```python
from build123d import *

# Parameters (mm, degrees)
F3_DEPTH        = 6
F3_COPIES_COUNT = 9


# Not quite as in the source:
# - a pattern or mirror of a feature is missing from the dataset's text; its kind, count and spacing are read off the source's solid


with BuildPart() as f1:
    # F0 (on Front) → F1 (revolve)
    with BuildSketch(Plane.XZ):
        Polygon((6, 0), (2.5, 0), (2, -2), (2, -10), (4.25, -10), (4.25, -4), (4.9, -4), (4.9, -2), (6, -2), align=None)
    revolve(axis=Axis((0, 0, -12.1953526796), (0, 0, -1)))

    # F2 (on face) → F3 (join, through all)
    with BuildSketch(Plane(origin=(0, 0, -10), x_dir=(1, 0, 0), z_dir=(0, 0, -1))):
        with BuildLine():
            ThreePointArc((-0.75, 4.1833001327), (0, 4.25), (0.75, 4.1833001327))
            Line((0.75, 4.1833001327), (0.75, 4.3833001327))
            Line((0.75, 4.3833001327), (-0.75, 4.3833001327))
            Line((-0.75, 4.3833001327), (-0.75, 4.1833001327))
        make_face()
    f3 = extrude(amount=-F3_DEPTH)

    # F3_copies: F3 ×9 about axis
    f3_copies_axis = Axis((0, 0, 0), (0, 0, 1))
    for i in range(1, F3_COPIES_COUNT):
        add(f3.rotate(f3_copies_axis, i * 360 / F3_COPIES_COUNT))


solid = f1.part
```
Can you work these out from the model? Positions are in its coordinate system, mm. A direction names the side the tool comes from. Coordinates: 2 decimals unless noted, no trailing zeros. Write each loop counter-clockwise with the first axis right and the second up, starting at its lowest first coordinate (ties: lowest second). Pieces come first, ordered by that corner, then holes. Notation, with made-up numbers: (-6.75, 79) - (-1.75, 79) arc R16 ccw to (-1.75, 86) - close; hole circle Ø10 at (64, 67.25). An arc over 180 degrees is marked (long way). Return JSON: item names as keys, results as strings.
Q1. If we section it at B-B (z = -1): Please give me the cut outline in (x, y), then the cut area to 3 significant figures.
Computed values:
{"outline": "circle Ø12 at (0, 0); hole circle Ø4.5 at (0, 0)", "area": "97.2 mm2"}
Q2. Thinking about a two-plate mould opening in X: for faces 4 (the cylindrical face through (1.46, -3.99, -6.96)), 5 (the cylindrical face through (4.184, 0.748, -6.958)), 6 (the flat face through (3, 0, 0)), which applies, +X half, -X half, draft (parallel to the pull), parting line (faces both ways), or undercut?
Computed values:
{"face 4": "undercut", "face 5": "+X half", "face 6": "draft"}
Q3. Please list where these lines run through material, in increasing order: L1, parallel to Y at x = 0, z = -4.5; L2, parallel to Z at x = -2.75, y = -4.5; L3, parallel to X at y = 1.5, z = -4.25. Write a range as from..to.
Computed values:
{"L1": "y = -4.38..-2, 2..4.25", "L2": "z = -2..0", "L3": "x = -4.1..-1.32, 1.32..4.1"}
Q4. If we section it at C-C (y = 5.25): Please give me the cut outline in (x, z), then the cut area to 3 significant figures.
Computed values:
{"outline": "(-2.9, -2) - (2.9, -2) - (2.9, 0) - (-2.9, 0) - close", "area": "11.6 mm2"}
Q5. I'm going to push flat-ended pins straight in: pin 1 Ø6 at (x, z) = (-2, -7.5) entering from +Y; pin 2 Ø1.6 at (x, z) = (0, -7.5) entering from -Y; pin 3 Ø3 at (x, y) = (0, 0) entering from -Z; pin 4 Ø2 at (y, z) = (2.5, -2) entering from +X. Where does each tip first touch, or does it pass through?
Computed values:
{"pin 1": "stops at y = 4.38", "pin 2": "stops at y = -4.38", "pin 3": "passes through", "pin 4": "stops at x = 5.81"}
Q6. On a 3-axis mill with a long thin cutter (end or side, diameter ignored), from which of +Z, -Z, +X, -X, +Y, -Y can I reach the whole of each face in a straight line? I mean faces 1 (the cylindrical face through (-4.187, 0.728, -6.958)), 2 (the cylindrical face through (-1.062, 4.783, -2.986)), 3 (the flat face through (4.32, -0.75, -7.04)). Say none if no direction works.
Computed values:
{"face 1": "-Z, -X", "face 2": "-Z", "face 3": "-Z, +X, -Y"}
Q7. If we section it at A-A (x = 0): Please give me the cut outline in (y, z).
Computed values:
{"outline": "(-6, -2) - (-4.9, -2) - (-4.9, -4) - (-4.38, -4) - (-4.38, -10) - (-2, -10) - (-2, -2) - (-2.5, 0) - (-6, 0) - close; (2, -10) - (4.25, -10) - (4.25, -4) - (4.9, -4) - (4.9, -2) - (6, -2) - (6, 0) - (2.5, 0) - (2, -2) - close"}
